Part model, mm, in its own coordinate system. Face numbers are marked on the shaded views. A direction names the side the tool comes from. Give positions to 0.01 mm unless a question says otherwise; leave off trailing zeros. Order: outer loops, then holes, each group sorted by start corner. A loop starts at its lowest first (then second) coordinate and runs counter-clockwise, first axis right, second up. Notation, with made-up numbers: (59, 13.25) - (103, 13.25) arc R18 ccw to (103, 36.25) - close; hole circle Ø3 at (38, -9). An arc over 180 degrees is marked (long way). One line per item, written item: value.
```python
from build123d import *

# Parameters (mm, degrees)
CROQUIS1_W              = 48
CROQUIS1_H              = 48
SALIENTE_EXTRUIR1_DEPTH = 5
CORTAR_EXTRUIR1_DEPTH   = 11
CORTAR_EXTRUIR1_DRAFT   = 7
CROQUIS3_W              = 48
CROQUIS3_H              = 48
SALIENTE_EXTRUIR2_DEPTH = 4


with BuildPart() as part:
    # Croquis1 → Saliente-Extruir1 (new, symmetric)
    with BuildSketch(Plane.XY):
        Rectangle(CROQUIS1_W, CROQUIS1_H)
    extrude(amount=SALIENTE_EXTRUIR1_DEPTH, both=True)


with BuildPart() as cortar_extruir1_tool:
    # Croquis2 → Cortar-Extruir1 (with draft: the straight prism first)
    with BuildSketch(Plane.XY.offset(5)):
        with BuildLine():
            ThreePointArc((-9.604686356, 8), (-11.421696131, -5.078863799), (-0.493320879, -12.490261587))
            Line((-0.493320879, -12.490261587), (9.604686356, 5))
            Line((9.604686356, 5), (9.604686356, 8))
            Line((9.604686356, 8), (-9.604686356, 8))
        make_face()
    extrude(amount=-CORTAR_EXTRUIR1_DEPTH)
    # Cortar-Extruir1: the draft: its side faces are tilted about the plane it starts from
    cortar_extruir1_sides = [cortar_extruir1_tool.faces().sort_by_distance(p)[0] for p in [
        (4.555682738, -3.745130793, -0.5),
        (9.604686356, 6.5, -0.5),
        (0, 8, -0.5),
        (-11.421696131, -5.078863799, -0.5),
    ]]
    draft(cortar_extruir1_sides, Plane.XY.offset(5), CORTAR_EXTRUIR1_DRAFT)


with BuildPart() as part_1:
    add(part.part)

    # Cortar-Extruir1: cut by cortar_extruir1_tool
    add(cortar_extruir1_tool.part, mode=Mode.SUBTRACT)

    # Croquis3 → Saliente-Extruir2 (add)
    with BuildSketch(Plane.XY.offset(5)):
        Rectangle(CROQUIS3_W, CROQUIS3_H)
        with BuildLine():
            Line((9.604686356, 8), (9.604686356, 5))
            Line((9.604686356, 5), (-0.493320879, -12.490261587))
            ThreePointArc((-0.493320879, -12.490261587), (-11.421696131, -5.078863799), (-9.604686356, 8))
            Line((-9.604686356, 8), (9.604686356, 8))
        make_face(mode=Mode.SUBTRACT)
    extrude(amount=SALIENTE_EXTRUIR2_DEPTH)


solid = part_1.part
```
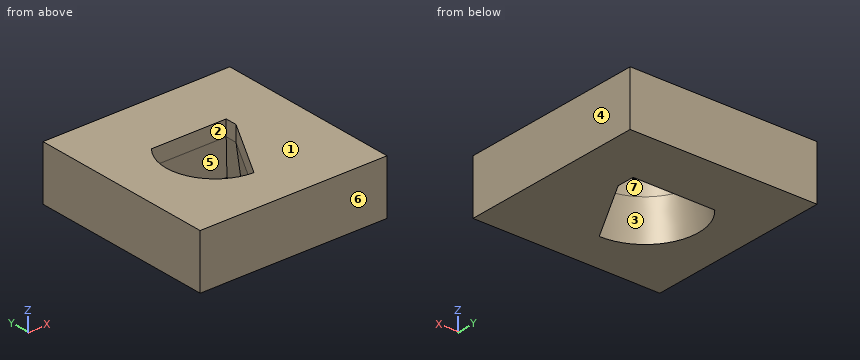
1) Which spindle directions (+Z, -Z, +X, -X, +Y, -Y) get a long thin tool onto all of the face, cutting with end or side? Do the marked faces 5, 6 and 7. Say none if no direction does.
Outcome:
face 5: -Z
face 6: +Z, -Z, +X, -X, -Y
face 7: +Z, -Z
2) Mould opens along X. For the marked faces 1, 2, 3 and 4 say: released by +X, released by -X, zero draft, split by the parting line, or undercut.
Outcome:
face 1: zero draft
face 2: undercut
face 3: undercut
face 4: released by +X
3) Cut at C-C, the plane z = -2.5. Give the cut face in (x, y), then the cut area to 3 significant figures.
Outcome:
outline: (-24, -24) - (24, -24) - (24, 24) - (-24, 24) - close; hole (-10.03, 8.92) arc R13.42 ccw to (0.03, -13.42) - (10.53, 4.75) - (10.53, 8.92) - close
area: 1,910 mm^2
4) Cut at B-B, the plane y = 0. Give the cut face in (x, z).
Outcome:
outline: (-24, -5) - (-13.73, -5) - (-12.5, 5) - (-12.5, 9) - (-24, 9) - close; (6.72, 5) - (8.14, -5) - (24, -5) - (24, 9) - (6.72, 9) - close
5) Cut at D-D, the plane z = 3.25. Give the cut face in (x, y), then the cut area to 3 significant figures.
Outcome:
outline: (-24, -24) - (24, -24) - (24, 24) - (-24, 24) - close; hole (-9.7, 8.21) arc R12.71 ccw to (-0.37, -12.71) - (9.82, 4.94) - (9.82, 8.21) - close
area: 1,960 mm^2
6) Cut at A-A, the plane x = 1. Give the cut face in (y, z), then the cut area to 3 significant figures.
Outcome:
outline: (-24, -5) - (-12.36, -5) - (-9.9, 5) - (-9.9, 9) - (-24, 9) - close; (8, 5) - (9.23, -5) - (24, -5) - (24, 9) - (8, 9) - close
area: 403 mm^2
7) Drill centre lines: line 1 along X through (y, z) = (0, 2.5); line 2 along Y through (x, z) = (-10, 4.25); line 3 along Y through (x, z) = (7, 0). Where is each one in solid material? Low to high. Write a range as from..to.
Outcome:
line 1: x = -24..-12.81, 7.07..24
line 2: y = -24..-7.65, 7.65..24
line 3: y = -24..-0.74, 8.61..24
